Input: part model. Units: mm. Frame: model coordinates. A direction names the side the tool comes from. Give positions to 0.01 mm unless a question says otherwise; leave off trailing zeros. Order: outer loops, then holes, each group sorted by start corner. A loop starts at its lowest first (then second) coordinate and runs counter-clockwise, first axis right, second up.
Autodesk Inventor part; units mm, degrees
ref_plane "YZ Plane" through (0, 0, 0) normal (1, 0, 0) x (0, 1, 0)
ref_plane "XZ Plane" through (0, 0, 0) normal (0, 1, 0) x (-1, 0, 0)
ref_plane "XY Plane" through (0, 0, 0) normal (0, 0, 1) x (1, 0, 0)
sketch "Body Outline" plane through (0, 0, 0) normal (0, 0, 1) x (1, 0, 0)
  line L0 (0, 0) -> (31, 0)
  line L1 (31, 0) -> (32.6381, -1.6381)
  line L2 (0, 0) -> (0, -9.5)
  line L3 (0, -9.5) -> (25, -9.5)
  line L4 (25, -9.5) -> (25, -17.6949)
  arc A0 (126.2645, -39.2876) -> (32.6381, -1.6381) centre (12, -188.2) ccw
  arc A1 (116.0982, -52.5366) -> (25, -17.6949) centre (12, -188.2) ccw
  line L5 (116.0982, -52.5366) -> (126.2645, -39.2876)
  dimension "d0" = 45
  dimension "d1" = 0
  dimension "d2" = 0
  dimension "d3" = 9.5
  dimension "d4" = 171
  dimension "d5" = 187.7
  dimension "d6" = 37.5
  dimension "d7" = 12
  dimension "d8" = 188.2
  dimension "d9" = 25
  dimension "d10" = 31
extrude "Body" add sketch "Body Outline" along normal mid plane 12.7
sketch "Dowel Pin Hole Positions" plane through (0, 0, 6.35) normal (0, 1, 0) x (1, 0, 0)
  line L0 (0, 12.7) -> (0, 0)
  point P0 (0, 6.35)
  point P1 (4, 6.35)
  point P2 (20, 6.35)
  dimension "d13" = 0
  dimension "d14" = 4
  dimension "d15" = 0
  dimension "d16" = 20
hole "Dowel Pin Holes" at (4, 0, 0) at (20, 0, 0) direction (0, -1, 0) diameter 2 end through all counterbore diameter 3.1 counterbore depth 7
sketch "Fastening Hole Position" plane through (0, 0, 6.35) normal (0, 1, 0) x (1, 0, 0)
  line L0 (0, 12.7) -> (0, 0)
  point P0 (0, 6.35)
  point P1 (12, 6.35)
  dimension "d24" = 0
  dimension "d25" = 12
hole "Fastening Hole" at (12, 0, 0) direction (0, -1, 0) diameter 8.1 end through all
sketch "Thumbscrew Cutout Outline" plane through (0, 0, 6.35) normal (0, 0, 1) x (1, 0, 0)
  arc A0 (126.2645, -39.2876) -> (32.6381, -1.6381) centre (12, -188.2) ccw
  line L0 (54.964, -27.8563) -> (60.5803, -6.8957) construction
  line L1 (0, 0) -> (0, -9.5)
  arc A1 (60.5803, -6.8957) -> (28.3591, -1.2143) centre (12, -188.2) ccw construction
  line L2 (12, -188.2) -> (28.3591, -1.2143) construction
  line L3 (12, -188.2) -> (60.5803, -6.8957) construction
  arc A2 (54.964, -27.8563) -> (26.4679, -22.8317) centre (12, -188.2) ccw construction
  line L4 (12, -188.2) -> (26.4679, -22.8317) construction
  line L5 (12, -188.2) -> (54.964, -27.8563) construction
  circle A3 centre (60.5803, -6.8957) radius 4
  dimension "d50" = 15
  dimension "d51" = 10
  dimension "d52" = 10
  dimension "d53" = 166
  dimension "d54" = 187.7
  dimension "d67" = 8
extrude "Thumbscrew Cutout" cut sketch "Thumbscrew Cutout Outline" against normal through all
pattern_circular "Thumbscrew Cutout Pattern" count 3 over 15 about axis through (12, -188.2, 0) along (0, 0, -1) of "Thumbscrew Cutout"
fillet "Body Fillet" radius 1 6 edges at (56.7058, -5.9017, 0) (64.4328, -7.9721, 0) (80.1181, -13.2965, 0) (87.5087, -16.3578, 0) (102.3648, -23.6841, 0) (109.2926, -27.6838, 0)
fillet "Body Fillet" radius 3 2 edges at (25, -9.5, 0) (25, -17.6949, 0)
fillet "Body Fillet" radius 7 2 edges at (126.2645, -39.2876, 0) (116.0982, -52.5366, 0)
equation "\"d54\" = d5"
properties part number "Arm Simplified" material "Aluminum 6061"
1) First-contact query: P1, Ø1.8, axis at x = 20, z = 0, coming from the +Y side; P2, Ø1.2, axis at y = -14, z = 2, coming from the -X side; P3, Ø2, axis at y = -12, z = 2, coming from the -X side; P4, Ø1, axis at x = 85, z = 2.5, coming from the -Y side. Flat tips, straight axial feed; report the tip coordinate or a pass-through.
2) Reachability of faces 4 (the face through (8, -9.5, 3)), 5 (the face through (44.13, -3.27, -0.09)), 6 (the face through (2.463, -3.549, -0.202)) from +Z, -Z, +X, -X, +Y, -Y: full face, straight path, thin tool, end or side. Return the list, or none.
3) Cut plane A-A (x = 60). Return the cut outline in (y, z), then the cut area to 3 significant figures.
4) Cut plane B-B (y = -22). Return the cut outline in (x, z).
5) Pull-direction query (X, two-part tool) for faces 1 (the face through (121.087, -46.036, -0.089)), 2 (the face through (82.229, -18.454, 0.089)), 3 (the face through (0, -5, 0)); classes: pulls with the +X half, pulls with the -X half, needs draft (parallel to the pull), parting line crosses it, or undercut.
6) Line query: probe 1 along Z at (x, y) = (20, -8); probe 2 along X at (y, z) = (-7.45, 0); probe 3 along Y at (x, z) = (19.5, 1). Output: solid intervals per line, ascending.
Geometry says:
1. P1: passes through
1. P2: stops at x = 25
1. P3: stops at x = 24.6
1. P4: stops at y = -33.8
2. face 4: +Z, -Z, -X, -Y
2. face 5: +Z, -Z, +X, +Y
2. face 6: +Y
3. outline: (-24.08, -6.35) - (-10.85, -6.35) - (-10.85, 6.35) - (-24.08, 6.35) - close
3. area: 168 mm2
4. outline: (52.23, -6.35) - (99.23, -6.35) - (99.23, 6.35) - (52.23, 6.35) - close
5. face 1: pulls with the +X half
5. face 2: undercut
5. face 3: pulls with the -X half
6. probe 1: z = -6.35 to -1, 1 to 6.35
6. probe 2: x = 0 to 3, 5 to 7.95, 16.05 to 19, 21 to 56.62
6. probe 3: y = -9.5 to -7
